CAD build for the part. Positions are in the model's coordinates, mm. A direction names the side the tool comes from. Round coordinates to 2 decimals unless told otherwise and drop trailing zeros. Write each loop counter-clockwise with the first axis right and the second up, starting at its lowest first coordinate (ties: lowest second). Pieces come first, ordered by that corner, then holes. Notation, with made-up numbers: (9, -19.5) -> (16, -19.5) arc R15 cw to (16, 7.5) -> close; hole circle Ø3 at (43.25, 33). An arc over 180 degrees is marked (long way). Answer in a Markdown table with one row per item. Add a question column.
```python
from build123d import *

# Parameters (mm, degrees)
SKETCH1_W           = 199.9
SKETCH1_H           = 200
BOSS_EXTRUDE1_DEPTH = 20
SHELL1_T            = -2
SKETCH2_R           = 6
CUT_EXTRUDE1_DEPTH  = 20
SKETCH3_W           = 20
SKETCH3_H           = 8
BOSS_EXTRUDE2_DEPTH = 3
RIB1_REACH          = 156.029
SKETCH5_WALL_W      = 317.868701922
SKETCH5_WALL_H      = 2
SKETCH6_R           = 1.5
BOSS_EXTRUDE3_DEPTH = 3
CUT_EXTRUDE2_DEPTH  = 154.460100678
FILLET1_R           = 2


with BuildPart() as part:
    # Sketch1 → Boss-Extrude1 (new body)
    with BuildSketch(Plane(origin=(0, 0, 0), x_dir=(1, 0, 0), z_dir=(0, 1, 0))):
        Rectangle(SKETCH1_W, SKETCH1_H)
    extrude(amount=BOSS_EXTRUDE1_DEPTH)

    # Shell1
    shell1_openings = [part.faces().sort_by_distance(p)[0] for p in [
        (0, 20, 0),
    ]]
    offset(amount=SHELL1_T, openings=shell1_openings, kind=Kind.INTERSECTION)

    # Sketch2 → Cut-Extrude1 (cut)
    with BuildSketch(Plane.XY.offset(100)):
        with Locations((84.95, 10)):
            Circle(SKETCH2_R)
    extrude(amount=-CUT_EXTRUDE1_DEPTH, mode=Mode.SUBTRACT)

    # Sketch3 → Boss-Extrude2 (add)
    with BuildSketch(Plane(origin=(0, 20, 0), x_dir=(1, 0, 0), z_dir=(0, 1, 0))):
        with Locations((0, -102)):
            Rectangle(SKETCH3_W, SKETCH3_H)
    extrude(amount=-BOSS_EXTRUDE2_DEPTH)

    # Sketch5 wall → Rib1 (add, up to next)
    with BuildSketch(Plane(origin=(-10, 14.5, 103), x_dir=(0, -0.640184399664, -0.768221279597), z_dir=(0, -0.768221279597, 0.640184399664)), mode=Mode.PRIVATE) as rib1_sk1:
        with Locations((0, 1)):
            Rectangle(SKETCH5_WALL_W, SKETCH5_WALL_H)
    rib1_tool1 = extrude(rib1_sk1.sketch, amount=-RIB1_REACH, mode=Mode.PRIVATE) - part.part
    rib1 = rib1_tool1.solids().sort_by_distance((-10, 14.5, 103))[0]
    add(rib1)

    # Mirror1: Rib1 across plane
    add(rib1.mirror(Plane(origin=(0, 0, 0), x_dir=(0, 0, 1), z_dir=(1, 0, 0))))

    # Sketch6 → Boss-Extrude3 (add)
    # profile 1 of 2: a face of its own
    with BuildSketch(Plane.XY.offset(100)):
        with BuildLine():
            Line((-104.95, 15), (-99.95, 15))
            Line((-99.95, 15), (-99.95, 5))
            Line((-99.95, 5), (-104.95, 5))
            ThreePointArc((-104.95, 5), (-109.95, 10), (-104.95, 15))
        make_face()
        with Locations((-104.95, 10)):
            Circle(SKETCH6_R, mode=Mode.SUBTRACT)
    # profile 2 of 2: a face of its own
    with BuildSketch(Plane.XY.offset(100)):
        with BuildLine():
            Line((104.95, 15), (99.95, 15))
            Line((99.95, 15), (99.95, 5))
            Line((99.95, 5), (104.95, 5))
            ThreePointArc((104.95, 5), (109.95, 10), (104.95, 15))
        make_face()
        with Locations(Location((104.95, 10, 0), (0, 0, 180))):
            Circle(SKETCH6_R, mode=Mode.SUBTRACT)
    extrude(amount=-BOSS_EXTRUDE3_DEPTH)

    # Sketch7 → Cut-Extrude2 (cut, through all)
    with BuildSketch(Plane(origin=(0, 15, 0), x_dir=(1, 0, 0), z_dir=(0, 1, 0))):
        with BuildLine():
            Line((105, -100), (109.95, -100))
            Line((109.95, -100), (109.95, -98.688929738))
            ThreePointArc((109.95, -98.688929738), (107.560342029, -99.666677231), (105, -100))
        make_face()
    extrude(amount=-CUT_EXTRUDE2_DEPTH, mode=Mode.SUBTRACT)

    # Fillet1
    fillet1_edges = [part.edges().sort_by_distance(p)[0] for p in [
        (-99.95, 10, 97),
        (-99.95, 15, 98.5),
        (-99.95, 5, 98.5),
        (99.95, 10, 97),
        (99.95, 5, 98.5),
        (99.95, 15, 98.5),
    ]]
    fillet(fillet1_edges, radius=FILLET1_R)


solid = part.part
```
Item 1: Saw through at B-B on z = -51. Give the cut face in (x, y).
Item 2: Tool access for faces 5 (the flat face through (10, 17, 102)), 6 (the flat face through (-8, 16, 102)), 7 (the cylindrical face through (-109.95, 9.89, 98.52)), 8 (the flat face through (107, 10, 97)), 9 (the flat face through (-1, 11, -98)): list every direction of +Z, -Z, +X, -X, +Y, -Y with a clear straight run to the whole face (end or side of a thin tool).
Item 3: Saw through at C-C on x = -75.5. Give the cut face in (y, z), then the cut area to 3 significant figures.
Item 4: Two-plate mould, pull along X, no slides. Class faces 1 (the cylindrical face through (109.95, 9.89, 98.19)), 2 (the cylindrical face through (83.649, 4.143, 99.014)), 3 (the flat face through (-10, 17, 102)), 4 (the flat face through (8, 16, 102)): +X half, -X half, draft (parallel to the pull), parting line (faces both ways), or undercut.
Item 5: Drill centre lines: probe 1 along Z at (x, y) = (-70.5, 7.5); probe 2 along X at (y, z) = (13.5, -38.5); probe 3 along Y at (x, z) = (104.95, 98.4). Where is each one in solid material? Low to high.
Item 6: Saw through at A-A on x = 84.95. Give the cut face in (y, z).
Item 7: Pin check, flat tips, straight feed: pin 1 (10 mm diameter, centred on y = 6.5, z = 47, fed in from -X); pin 2 (1.8 mm diameter, centred on y = 17, z = 102, fed in from -X); pin 3 (3.5 mm diameter, centred on x = -103, z = 99, fed in from +Y). Stop position of each tip, or through.
Recorded:
| question | item | result |
|---|---|---|
| 1 | outline | (-99.95, 0) -> (99.95, 0) -> (99.95, 20) -> (97.95, 20) -> (97.95, 2) -> (-97.95, 2) -> (-97.95, 20) -> (-99.95, 20) -> close |
| 2 | face 5 | +Z, +X, +Y, -Y |
| 2 | face 6 | +Z, -Y |
| 2 | face 7 | +Z, -Z, -X |
| 2 | face 8 | -Z, +X, +Y, -Y |
| 2 | face 9 | +Y |
| 3 | outline | (0, -100) -> (20, -100) -> (20, -98) -> (2, -98) -> (2, 98) -> (20, 98) -> (20, 100) -> (0, 100) -> close |
| 3 | area | 472 mm2 |
| 4 | face 1 | +X half |
| 4 | face 2 | undercut |
| 4 | face 3 | -X half |
| 4 | face 4 | undercut |
| 5 | probe 1 | -100 to -98, 98 to 100 |
| 5 | probe 2 | -99.95 to -97.95, 97.95 to 99.95 |
| 5 | probe 3 | 5 to 8.5, 11.5 to 15 |
| 6 | outline | (0, -100) -> (20, -100) -> (20, -98) -> (2, -98) -> (2, 98) -> (4, 98) -> (4, 100) -> (0, 100) -> close; (16, 98) -> (20, 98) -> (20, 100) -> (16, 100) -> close |
| 7 | pin 1 | x = -99.95 |
| 7 | pin 2 | x = -10 |
| 7 | pin 3 | y = 15.13 |
